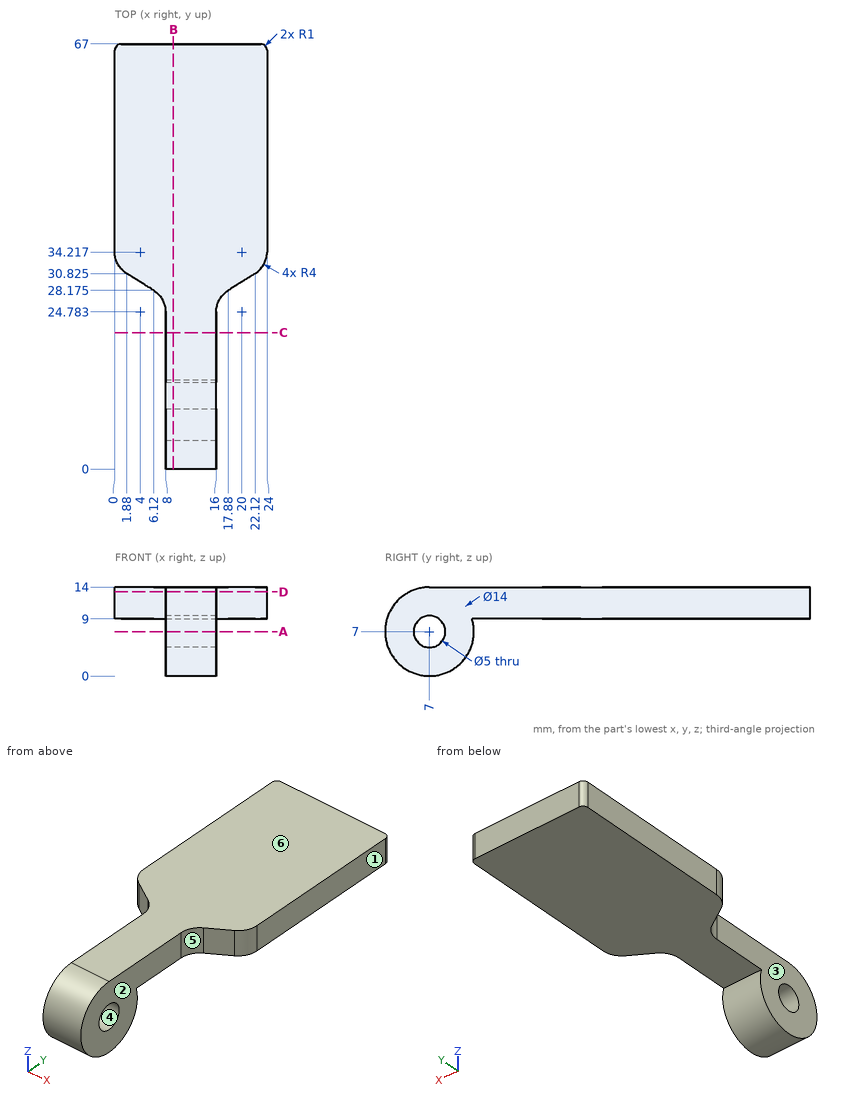
The drawing under review shows one solid part. Ordinate dimensions are in mm from its lowest x, y, z. A direction names the side the tool comes from. Round coordinates to 2 decimals unless told otherwise and drop trailing zeros. Order: outer loops, then holes, each group sorted by start corner. A loop starts at its lowest first (then second) coordinate and runs counter-clockwise, first axis right, second up. Notation, with made-up numbers: (44, 62) - (53, 62) arc R23 ccw to (53, 82) - close; hole circle Ø3 at (78, 81.5). An arc over 180 degrees is marked (long way). Return JSON: item names as keys, results as strings.
Q1. Machinability: for the marked faces 1, 2 and 3, which of the approach directions +Z, -Z, +X, -X, +Y, -Y give a long, thin tool a straight path to every point of the face, cutting with its end or side? Answer none if there is none.
Computed values:
{"face 1": "+Z, -Z, +X, +Y, -Y", "face 2": "+Z, -Z, +X, -Y", "face 3": "+Z, -Z, -X, -Y"}
Q2. Consider section C-C on y = 21.5. Write out the cut boundary in (x, z), plus the area to 3 significant figures.
Computed values:
{"outline": "(8, 9) - (16, 9) - (16, 14) - (8, 14) - close", "area": "40.0 mm2"}
Q3. Consider section A-A on z = 7. Write out the cut boundary in (x, y), plus the area to 3 significant figures.
Computed values:
{"outline": "(8, 0) - (16, 0) - (16, 4.5) - (8, 4.5) - close; (8, 9.5) - (16, 9.5) - (16, 14) - (8, 14) - close", "area": "72.0 mm2"}
Q4. Wall thickness on L1, parallel to Z at x = 14.25, y = 7; L2, parallel to Z at x = 16.5, y = 28.5: over which ranges is each line inside the solid? List them lowest first. Write a range as [from, to].
Computed values:
{"L1": "z = [0, 4.5], [9.5, 14]", "L2": "z = [9, 14]"}
Q5. The part is to be moulded in two halves that separate along Z. For the marked faces 4, 5 and 6, say which applies: pulls with the +Z half, pulls with the -Z half, needs draft (parallel to the pull), parting line crosses it, or undercut.
Computed values:
{"face 4": "undercut", "face 5": "needs draft", "face 6": "pulls with the +Z half"}
Q6. Consider section D-D on z = 13.25. Write out the cut boundary in (x, y) (3 decimals).
Computed values:
{"outline": "(0, 34.217) arc R4 ccw to (1.88, 30.825) - (6.12, 28.175) arc R4 cw to (8, 24.783) - (8, 3.848) - (16, 3.848) - (16, 24.783) arc R4 cw to (17.88, 28.175) - (22.12, 30.825) arc R4 ccw to (24, 34.217) - (24, 66) arc R1 ccw to (23, 67) - (1, 67) arc R1 ccw to (0, 66) - close"}
Q7. Consider section B-B on x = 9.25. Write out the cut boundary in (y, z), plus the area to 3 significant figures.
Computed values:
{"outline": "(7, 14) arc R7 ccw (long way) to (13.71, 9) - (67, 9) - (67, 14) - close; hole circle Ø5 at (7, 7)", "area": "410 mm2"}
Q8. For pin 1 Ø5 at (x, z) = (18, 10) entering from -Y; pin 2 Ø7 at (x, y) = (17.5, 31.5) entering from -Z; pin 3 Ø5 at (x, z) = (16.5, 2) entering from -Y; pin 4 Ø6 at (y, z) = (43.5, 8.5) entering from +X, all flat-tipped, find the tip position at first contact; note any pin that passes through.
Computed values:
{"pin 1": "stops at y = 0.16", "pin 2": "stops at z = 9", "pin 3": "stops at y = 0.48", "pin 4": "stops at x = 24"}
